Read the model definition and answer for the solid it produces. Units are mm, in the model's axes. Give positions to 0.01 mm unless a question says otherwise; leave off trailing zeros. Write each loop counter-clockwise with the first axis right and the second up, starting at its lowest first coordinate (ties: lowest second). Pieces come first, ordered by that corner, then holes. Notation, with made-up numbers: (73.5, 81) - (96.5, 81) arc R30 ccw to (96.5, 112) - close; hole circle Ø11 at (50, 71). An arc over 180 degrees is marked (long way). Use CSV: the item, a comma, the result in double quotes. Start each with the question number.
from build123d import *

# Parameters (mm, degrees)
CYLINDER002_R     = 2.5
CYLINDER002_DEPTH = 3
CYLINDER001_R     = 9
CYLINDER001_DEPTH = 3
CYLINDER003_R     = 2.5
CYLINDER003_DEPTH = 3
CYLINDER004_R     = 2.5
CYLINDER004_DEPTH = 3
CYLINDER005_R     = 2.5
CYLINDER005_DEPTH = 3
BOX002_W          = 35
BOX002_H          = 35
BOX002_DEPTH      = 3
FILLET002_R       = 1.5


with BuildPart() as cylinder002:
    # Cylinder002 → Cylinder002 (new body)
    with BuildSketch(Plane(origin=(10, 10, 0), x_dir=(1, 0, 0), z_dir=(0, 0, 1))):
        Circle(CYLINDER002_R)
    extrude(amount=CYLINDER002_DEPTH)


with BuildPart() as cylinder001:
    # Cylinder001 → Cylinder001 (new body)
    with BuildSketch(Plane(origin=(20, 20, 0), x_dir=(1, 0, 0), z_dir=(0, 0, 1))):
        Circle(CYLINDER001_R)
    extrude(amount=CYLINDER001_DEPTH)


with BuildPart() as cylinder003:
    # Cylinder003 → Cylinder003 (new body)
    with BuildSketch(Plane(origin=(30, 10, 0), x_dir=(1, 0, 0), z_dir=(0, 0, 1))):
        Circle(CYLINDER003_R)
    extrude(amount=CYLINDER003_DEPTH)


with BuildPart() as cylinder004:
    # Cylinder004 → Cylinder004 (new body)
    with BuildSketch(Plane(origin=(10, 30, 0), x_dir=(1, 0, 0), z_dir=(0, 0, 1))):
        Circle(CYLINDER004_R)
    extrude(amount=CYLINDER004_DEPTH)


with BuildPart() as cylinder005:
    # Cylinder005 → Cylinder005 (new body)
    with BuildSketch(Plane(origin=(30, 30, 0), x_dir=(1, 0, 0), z_dir=(0, 0, 1))):
        Circle(CYLINDER005_R)
    extrude(amount=CYLINDER005_DEPTH)


with BuildPart() as cut006:
    # Box002 → Box002 (new body)
    with BuildSketch(Plane(origin=(2.5, 2.5, 0), x_dir=(1, 0, 0), z_dir=(0, 0, 1))):
        with Locations((17.5, 17.5)):
            Rectangle(BOX002_W, BOX002_H)
    extrude(amount=BOX002_DEPTH)

    # Fillet002
    fillet002_edges = [cut006.edges().sort_by_distance(p)[0] for p in [
        (2.5, 2.5, 1.5),
        (2.5, 37.5, 1.5),
        (37.5, 2.5, 1.5),
        (37.5, 37.5, 1.5),
    ]]
    fillet(fillet002_edges, radius=FILLET002_R)

    # Cut002: cut Cylinder005
    add(cylinder005.part, mode=Mode.SUBTRACT)

    # Cut003: cut Cylinder004
    add(cylinder004.part, mode=Mode.SUBTRACT)

    # Cut004: cut Cylinder003
    add(cylinder003.part, mode=Mode.SUBTRACT)

    # Cut005: cut Cylinder001
    add(cylinder001.part, mode=Mode.SUBTRACT)

    # Cut006: cut Cylinder002
    add(cylinder002.part, mode=Mode.SUBTRACT)


solid = cut006.part
(1) The part is cut by section D-D on x = 20. Write down the section's boundary in (y, z).
(2) Given P1, Ø3, axis at x = 10, y = 30, coming from the +Z side, flat-ended and moving along its own axis, determine where the tip first touches the part or whether it passes through.
(3) For a pull along Y with two mould halves and no side action, classify faces 1 (the face through (28.16, 31.69, 1.48)), 2 (the face through (37.05, 2.93, 1.52)), 3 (the face through (20, 37.5, 1)), 4 (the face through (9.46, 7.56, 1.48)) as pulls with the +Y half, pulls with the -Y half, needs draft (parallel to the pull), parting line crosses it, or undercut.
(4) The part is cut by section C-C on z = 2.1. Write down the section's boundary in (x, y), plus the area to 3 significant figures.
(5) Consider probe 1 along Y at (x, z) = (10, 0.6); probe 2 along Y at (x, z) = (30.5, 1.4); probe 3 along X at (y, z) = (13.5, 1.1). Determine where each line is inside the solid, lowest interval first.
(6) The part is cut by section A-A on x = 30. Write down the section's boundary in (y, z), plus the area to 3 significant figures.
Reported:
1,outline,"(2.5, 0) - (11, 0) - (11, 3) - (2.5, 3) - close; (29, 0) - (37.5, 0) - (37.5, 3) - (29, 3) - close"
2,P1,"through"
3,face 1,"undercut"
3,face 2,"pulls with the -Y half"
3,face 3,"pulls with the +Y half"
3,face 4,"undercut"
4,outline,"(2.5, 4) arc R1.5 ccw to (4, 2.5) - (36, 2.5) arc R1.5 ccw to (37.5, 4) - (37.5, 36) arc R1.5 ccw to (36, 37.5) - (4, 37.5) arc R1.5 ccw to (2.5, 36) - close; hole circle Ø5 at (10, 10); hole circle Ø5 at (10, 30); hole circle Ø18 at (20, 20); hole circle Ø5 at (30, 10); hole circle Ø5 at (30, 30)"
4,area,"890 mm²"
5,probe 1,"2.5 to 7.5, 12.5 to 27.5, 32.5 to 37.5"
5,probe 2,"2.5 to 7.55, 12.45 to 27.55, 32.45 to 37.5"
5,probe 3,"2.5 to 13.78, 26.22 to 37.5"
6,outline,"(2.5, 0) - (7.5, 0) - (7.5, 3) - (2.5, 3) - close; (12.5, 0) - (27.5, 0) - (27.5, 3) - (12.5, 3) - close; (32.5, 0) - (37.5, 0) - (37.5, 3) - (32.5, 3) - close"
6,area,"75.0 mm²"
